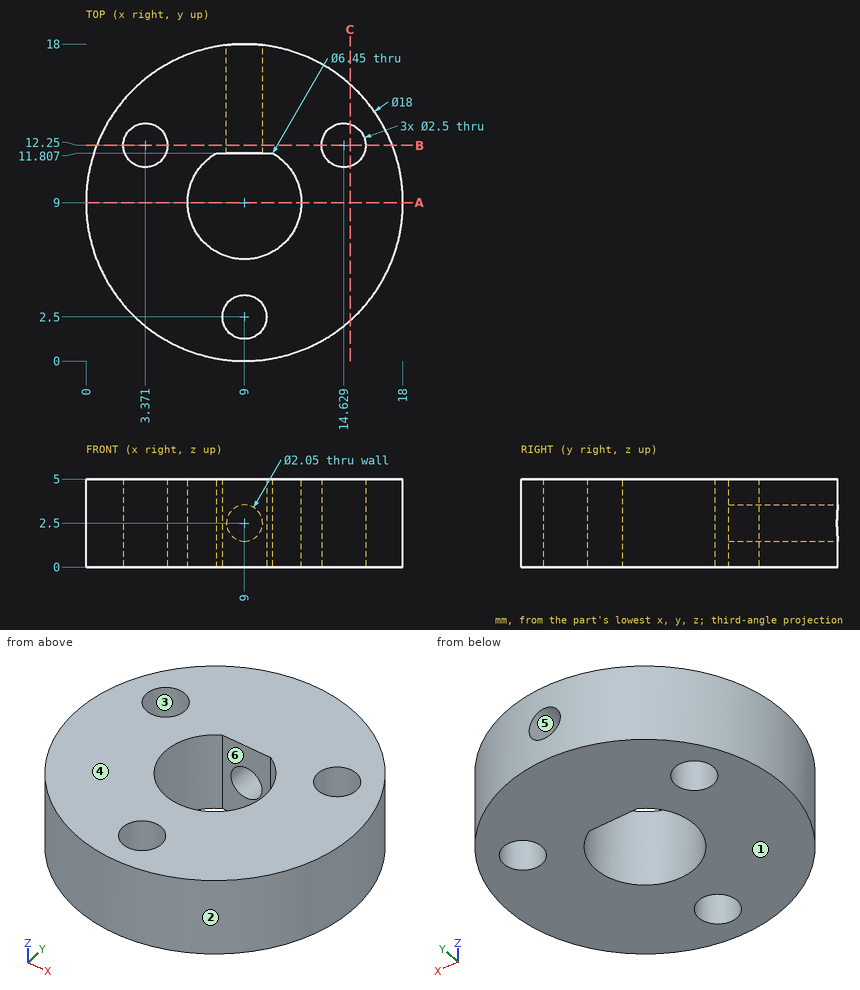
Geometry check sheet. Reference: drawing and pictorial views, mm from the part's lowest x, y, z. A direction names the side the tool comes from. Coordinates: 2 decimals unless noted, no trailing zeros. Write each loop counter-clockwise with the first axis right and the second up, starting at its lowest first coordinate (ties: lowest second). Pieces come first, ordered by that corner, then holes. Notation, with made-up numbers: M 0,16 L 56,16 A19 cw 56,36 Z; hole C -30,78 d6. An arc over 180 degrees is marked long. Write item = value, one per line. Start each with the question number.
1. Sectioned sample at A-A (y = 9). Record the cut outline in (x, z) (3 decimals).
2. Go/stop test with flat-tipped pins: pin 1 (1 mm diameter, centred on x = 11, y = 10, fed in from -Z); pin 2 (1.8 mm diameter, centred on x = 9, z = 2.5, fed in from +Y). Record where each tip stops, or that it passes through.
3. Sectioned sample at B-B (y = 12.25). State how many separate pieces and enclosed holes the cut face has.
4. Tool access check on the marked faces 4, 5 and 6. Record the directions out of +Z, -Z, +X, -X, +Y, -Y that give a thin tool (end or side, any length) a straight path to the whole face; none if there is none.
5. Thickness scan on probe 1 along Y at (x, z) = (6.5, 0.75) (1 decimal); probe 2 along Z at (x, y) = (8.5, 15.75) (1 decimal); probe 3 along Y at (x, z) = (4.25, 4.45) (1 decimal). Record the ranges inside material, lowest first.
6. Mould release check, pull along Y, two halves, no side actions. Record for the marked faces 1, 2 and 3: pulls with the +Y half, pulls with the -Y half, needs draft (parallel to the pull), parting line crosses it, or undercut.
7. Sectioned sample at C-C (x = 15). Record the cut outline in (y, z).
The answers:
q1.outline = M 0,0 L 5.775,0 L 5.775,5 L 0,5 Z; M 12.225,0 L 18,0 L 18,5 L 12.225,5 Z
q2.pin_1 = through
q2.pin_2 = 5.9
q3.separate_pieces = 3
q3.enclosed_holes = 1
q4.face_4 = +Z, +X, -X, +Y, -Y
q4.face_5 = +Y
q4.face_6 = +Z, -Z
q5.probe_1 = 0.4 to 7, 11 to 17.6
q5.probe_2 = 0 to 1.6, 3.4 to 5
q5.probe_3 = 1.4 to 11.4, 13.1 to 16.6
q6.face_1 = needs draft
q6.face_2 = parting line crosses it
q6.face_3 = undercut
q7.outline = M 2.29,0 L 11.06,0 L 11.06,5 L 2.29,5 Z; M 13.44,0 L 15.71,0 L 15.71,5 L 13.44,5 Z
